Part model, mm, in its own coordinate system. Face numbers are marked on the shaded views. A direction names the side the tool comes from. Round coordinates to 2 decimals unless told otherwise and drop trailing zeros. Order: outer loops, then holes, each group sorted by start corner. A loop starts at its lowest first (then second) coordinate and runs counter-clockwise, first axis right, second up. Notation, with made-up numbers: (60.5, 37) -> (72.5, 37) arc R16 cw to (72.5, 45) -> close; hole circle Ø5 at (1.5, 76.5). An arc over 180 degrees is marked (long way). Use CSV: the item, a comma, the result in double quotes.
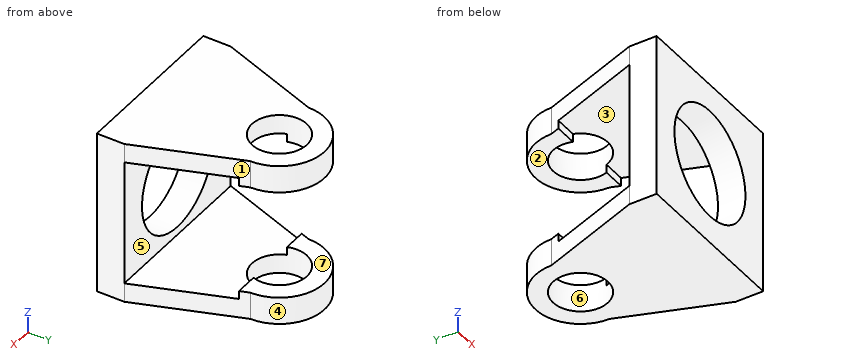
```python
from build123d import *

# Parameters (mm, degrees)
SKETCH1_W           = 30
SKETCH1_H           = 30
BOSS_EXTRUDE1_DEPTH = 5
BOSS_EXTRUDE2_DEPTH = 5
BOSS_EXTRUDE3_START = -5
BOSS_EXTRUDE3_DEPTH = 5
SKETCH6_R           = 5
CUT_EXTRUDE1_DEPTH  = 38
SKETCH7_R           = 10
CUT_EXTRUDE2_DEPTH  = 5
SKETCH8_W           = 23.0008229
SKETCH8_H           = 16.927991413
CUT_EXTRUDE3_DEPTH  = 30


with BuildPart() as part:
    # Sketch1 → Boss-Extrude1 (new body)
    with BuildSketch(Plane(origin=(0, 0, 0), x_dir=(1, 0, 0), z_dir=(0, 1, 0))):
        Rectangle(SKETCH1_W, SKETCH1_H)
    extrude(amount=BOSS_EXTRUDE1_DEPTH)

    # Sketch3 → Boss-Extrude2 (add)
    with BuildSketch(Plane.XY.offset(15)):
        with BuildLine():
            Line((-15, 5), (-8.229784678, 23.601013721))
            ThreePointArc((-8.229784678, 23.601013721), (0, 31.830798399), (8.229784678, 23.601013721))
            Line((8.229784678, 23.601013721), (15, 5))
            Line((15, 5), (-15, 5))
        make_face()
    extrude(amount=-BOSS_EXTRUDE2_DEPTH)

    # Sketch5 → Boss-Extrude3 (add)
    with BuildSketch(Plane(origin=(0, 0, -15), x_dir=(-1, 0, 0), z_dir=(0, 0, -1)).offset(BOSS_EXTRUDE3_START)):
        with BuildLine():
            Line((-15, 5), (-8.229784678, 23.601013721))
            ThreePointArc((-8.229784678, 23.601013721), (0, 31.830798399), (8.229784678, 23.601013721))
            Line((8.229784678, 23.601013721), (15, 5))
            Line((15, 5), (-15, 5))
        make_face()
    extrude(amount=BOSS_EXTRUDE3_DEPTH)

    # Sketch6 → Cut-Extrude1 (cut)
    with BuildSketch(Plane(origin=(0, 0, -15), x_dir=(-1, 0, 0), z_dir=(0, 0, -1))):
        with Locations((0, 23.601013721)):
            Circle(SKETCH6_R)
    extrude(amount=-CUT_EXTRUDE1_DEPTH, mode=Mode.SUBTRACT)

    # Sketch7 → Cut-Extrude2 (cut)
    with BuildSketch(Plane.XZ):
        with Locations(Location((0, 0, 0), (0, 0, 270))):
            Circle(SKETCH7_R)
    extrude(amount=-CUT_EXTRUDE2_DEPTH, mode=Mode.SUBTRACT)

    # Sketch8 → Cut-Extrude3 (cut)
    with BuildSketch(Plane(origin=(15, 0, 0), x_dir=(0, 0, -1), z_dir=(1, 0, 0))):
        with Locations((0, 13.463995707)):
            Rectangle(SKETCH8_W, SKETCH8_H)
    extrude(amount=-CUT_EXTRUDE3_DEPTH, mode=Mode.SUBTRACT)


solid = part.part
```
(1) Probe probe 1 along X at (y, z) = (1.7, 0); probe 2 along Z at (x, y) = (9.75, 17); probe 3 along Y at (x, z) = (0, -13.6). List the from-to ranges inside material, lowest first. Write a range as [from, to].
Reply:
probe 1,"[-15, -10], [10, 15]"
probe 2,"[-15, -11.5], [11.5, 15]"
probe 3,"[0, 18.6], [28.6, 31.83]"
(2) Cut at A-A, the plane z = 0. Give the cut face in (x, y).
Reply:
outline,"(-15, 0) -> (-10, 0) -> (-10, 5) -> (-15, 5) -> close; (10, 0) -> (15, 0) -> (15, 5) -> (10, 5) -> close"
(3) Pull direction Y, two halves, no side cores. Call the marked faces 4, 5, 6 and 7: released by +Y, released by -Y, zero draft, split by the parting line, or undercut.
Reply:
face 4,"released by +Y"
face 5,"undercut"
face 6,"undercut"
face 7,"zero draft"
(4) Cut at C-C, the plane y = 2. Give the cut face in (x, z).
Reply:
outline,"(-15, -15) -> (15, -15) -> (15, 15) -> (-15, 15) -> close; hole circle Ø20 at (0, 0)"
(5) Cut at D-D, the plane z = 12.25. Give the cut face in (x, y), then the cut area to 3 significant figures.
Reply:
outline,"(-15, 0) -> (15, 0) -> (15, 5) -> (8.23, 23.6) arc R8.23 ccw to (-8.23, 23.6) -> (-15, 5) -> close; hole circle Ø10 at (0, 23.6)"
area,"610 mm2"
(6) Cut at B-B, the plane x = -9.5. Give the cut face in (y, z).
Reply:
outline,"(0, -15) -> (20.11, -15) -> (20.11, -11.5) -> (5, -11.5) -> (5, -3.12) -> (0, -3.12) -> close; (0, 3.12) -> (5, 3.12) -> (5, 11.5) -> (20.11, 11.5) -> (20.11, 15) -> (0, 15) -> close"
(7) Drop flat-ended pins along their axis: P1, Ø2, axis at x = -9, z = 2, coming from the +Y side; P2, Ø3, axis at y = 12.5, z = -11, coming from the +X side. Give the stop position or say it passes through.
Reply:
P1,"y = 5"
P2,"x = 12.78"
(8) Which spindle directions (+Z, -Z, +X, -X, +Y, -Y) get a long thin tool onto all of the face, cutting with end or side? Do the marked faces 1, 2 and 3. Say none if no direction does.
Reply:
face 1,"+Z, -Z, +X, +Y"
face 2,"+X, -X, +Y"
face 3,"+X, -X"
